Part model, mm, in its own coordinate system. Face numbers are marked on the shaded views. A direction names the side the tool comes from. Round coordinates to 2 decimals unless told otherwise and drop trailing zeros. Write each loop counter-clockwise with the first axis right and the second up, starting at its lowest first coordinate (ties: lowest second). Pieces come first, ordered by that corner, then holes. Notation, with made-up numbers: M 86.25,-31.5 L 132.25,-31.5 A25 cw 132.25,-18.5 Z; hole C -2,-3.5 d4. An arc over 180 degrees is marked long. Use a Markdown table: item, result. Add a question column.
1) Two-plate mould, pull along Y, no slides. Class the marked faces 4, 5 and 6: released by +Y, released by -Y, zero draft, split by the parting line, or undercut.
2) Wall check: probe 1 along Z at (x, y) = (-10.75, 13); probe 2 along Y at (x, z) = (9.25, 10); probe 3 along Y at (x, z) = (12.25, -13). Give the ranges that are in metal, low to high.
3) Slice it at B-B on y = 26.5. Write the cut outline in (x, z), plus the area to 3 significant figures.
4) Slice it at A-A on x = 11. Write the cut outline in (y, z).
5) Drop flat-ended pins along their axis: P1, Ø4.5, axis at x = -2, y = 7, coming from the -Z side; P2, Ø1.7, axis at x = 11, z = 16.5, coming from the +Y side; P3, Ø8.5, axis at x = -3.5, y = 20.5, coming from the +Z side. Give the stop position or say it passes through.
6) Which spindle directions (+Z, -Z, +X, -X, +Y, -Y) get a long thin tool onto all of the face, cutting with end or side? Do the marked faces 1, 2 and 3. Say none if no direction does.
7) Slice it at C-C on x = -2.75. Write the cut outline in (y, z).
Autodesk Inventor part; units mm, degrees
ref_plane "YZ Plane" through (0, 0, 0) normal (1, 0, 0) x (0, 1, 0)
ref_plane "XZ Plane" through (0, 0, 0) normal (0, 1, 0) x (-1, 0, 0)
ref_plane "XY Plane" through (0, 0, 0) normal (0, 0, 1) x (1, 0, 0)
sketch "Sketch1" plane through (0, 0, 0) normal (0, 1, 0) x (-1, 0, 0)
  line L0 (6.2884, 19.9233) -> (-5.9116, 19.9233)
  line L1 (-5.9116, 19.9233) -> (-5.9116, 12.6233)
  line L2 (-5.9116, 12.6233) -> (6.2884, 12.6233)
  line L3 (6.2884, 12.6233) -> (6.2884, 19.9233)
  point P0 (0, 0)
  dimension "d0" = 7.3
  dimension "d1" = 12.2
extrude "Extrusion1" add sketch "Sketch1" along normal blind 3
sketch "Sketch2" plane through (0, 3, 0) normal (0, 1, 0) x (1, 0, 0)
  line L0 (5.9116, -19.9233) -> (5.9116, -12.6233)
  line L1 (5.9116, -12.6233) -> (-6.2884, -12.6233)
  line L2 (-6.2884, -12.6233) -> (-6.2884, -19.9233)
  line L3 (-6.2884, -19.9233) -> (5.9116, -19.9233)
  line L4 (5.9116, -12.6233) -> (-6.2884, -12.6233)
  line L5 (-6.2884, -12.6233) -> (-6.2884, -14.1233)
  line L6 (-6.2884, -14.1233) -> (5.9116, -14.1233)
  line L7 (5.9116, -14.1233) -> (5.9116, -12.6233)
  point P0 (0, 0)
  point P1 (5.9116, -14.1233)
  dimension "d4" = 1.5
extrude "Extrusion2" add sketch "Sketch2" along normal blind 15.7 contours L6 L2 L1 L0
sketch "Sketch3" plane through (5.9116, 0, 12.6233) normal (0, 0, -1) x (-1, 0, 0)
  line L0 (0, 0) -> (12.2, 0)
  line L1 (12.2, 0) -> (12.2, 18.7)
  line L2 (0, 18.7) -> (12.2, 18.7)
  line L3 (0, 0) -> (0, 18.7)
  line L4 (0, 18.7) -> (12.2, 18.7)
  line L5 (12.2, 18.7) -> (12.2, 15.7)
  line L6 (12.2, 15.7) -> (0, 15.7)
  line L7 (0, 15.7) -> (0, 18.7)
  point P0 (5.9116, 0)
  point P1 (0, 15.7)
  dimension "d7" = 3
extrude "Extrusion3" add sketch "Sketch3" along normal blind 23.8 contours L3 L2 L1 L6
sketch "Sketch4" plane through (-6.2884, 15.7, 12.6233) normal (0, -1, 0) x (1, 0, 0)
  line L0 (0, 0) -> (12.2, 0)
  line L1 (0, 0) -> (0, -23.8)
  line L2 (12.2, -23.8) -> (0, -23.8)
  line L3 (12.2, 0) -> (12.2, -23.8)
  line L4 (12.2, -23.8) -> (0, -23.8)
  line L5 (0, -23.8) -> (0, -22.3)
  line L6 (0, -22.3) -> (12.2, -22.3)
  line L7 (12.2, -22.3) -> (12.2, -23.8)
  point P0 (6.2884, -12.6233)
  dimension "d10" = 1.5
extrude "Extrusion4" add sketch "Sketch4" along normal up to surface (15.7 mm away) contours L6 L3 L2 L1
sketch "Sketch5" plane through (5.9116, 0, -11.1767) normal (0, 0, -1) x (-1, 0, 0)
  line L0 (12.2, 18.7) -> (12.2, 0)
  line L1 (12.2, 18.7) -> (0, 18.7)
  line L2 (0, 18.7) -> (0, 0)
  line L3 (12.2, 0) -> (0, 0)
  line L4 (12.2, 0) -> (0, 0)
  line L5 (0, 0) -> (0, 3)
  line L6 (0, 3) -> (12.2, 3)
  line L7 (12.2, 3) -> (12.2, 0)
  point P0 (5.9116, 0)
  dimension "d13" = 3
extrude "Extrusion5" add sketch "Sketch5" along normal blind 5.8 contours L0 L3 L2 L6
sketch "Sketch6" plane through (0, 0, 0) normal (0, -1, 0) x (1, 0, 0)
  arc A0 (-0.7384, -2.4741) -> (0.3616, -2.4741) centre (-0.1884, -3.4267) ccw construction
  circle A1 centre (-0.1884, -3.4267) radius 1.1 construction
  arc A2 (0.3616, -32.1794) -> (-0.7384, -32.1794) centre (-0.1884, -31.2267) ccw
  circle A3 centre (-0.1884, -31.2267) radius 1.5
  circle A4 centre (-0.1884, -3.4267) radius 1.5
  point P0 (0, 0)
  dimension "d16" = 3
  dimension "d17" = 3
extrude "Extrusion6" cut sketch "Sketch6" against normal up to surface (3 mm away)
sketch "Sketch8" plane through (5.9116, 0, 19.9233) normal (1, 0, 0) x (0, 0, -1)
  line L0 (0, 0) -> (7.3, 0)
  line L1 (7.3, 0) -> (7.3, 15.7)
  line L2 (7.3, 15.7) -> (29.6, 15.7)
  line L3 (29.6, 15.7) -> (29.6, 0)
  line L4 (36.9, 0) -> (29.6, 0)
  line L5 (36.9, 3) -> (36.9, 0)
  line L6 (31.1, 3) -> (36.9, 3)
  line L7 (31.1, 18.7) -> (31.1, 3)
  line L8 (5.8, 18.7) -> (31.1, 18.7)
  line L9 (5.8, 3) -> (5.8, 18.7)
  line L10 (0, 3) -> (5.8, 3)
  line L11 (0, 0) -> (0, 3)
  line L12 (0, 0) -> (36.9, 0)
  line L13 (36.9, 0) -> (36.9, 6)
  line L14 (36.9, 6) -> (0, 6)
  line L15 (0, 6) -> (0, 0)
  point P0 (19.9233, 0)
  dimension "d22" = 6
extrude "Extrusion8" add sketch "Sketch8" along normal blind 8 contours L11 L10 L9 L14 L1 L0 | L1 L14 L3 L12 | L15 L14 L9 L10 | L3 L14 L7 L6 L5 L4 | L14 L13 L6 L7
sketch "Sketch9" plane through (-6.2884, 0, 12.6233) normal (-1, 0, 0) x (0, 0, 1)
  line L0 (-29.6, 6) -> (7.3, 6)
  line L1 (7.3, 6) -> (7.3, 0)
  line L2 (7.3, 0) -> (-29.6, 0)
  line L3 (-29.6, 0) -> (-29.6, 6)
  point P0 (-12.6233, 0)
  point P1 (7.3, 6)
  point P2 (-29.6, 0)
extrude "Extrusion9" add sketch "Sketch9" along normal blind 8
sketch "Sketch10" plane through (13.9116, 0, 19.9233) normal (1, 0, 0) x (0, 0, -1)
  line L0 (0, 6) -> (0, 0)
  line L1 (0, 0) -> (36.9, 0)
  line L2 (36.9, 0) -> (36.9, 6)
  line L3 (36.9, 6) -> (0, 6)
  line L4 (0, 6) -> (36.9, 0) construction
  line L5 (36.9, 6) -> (0, 0) construction
  circle A0 centre (18.45, 3) radius 1.5
  point P0 (19.9233, 0)
  dimension "d27" = 3
extrude "Extrusion10" cut sketch "Sketch10" against normal blind 8 contours A0
sketch "Sketch11" plane through (0, 18.7, 0) normal (0, 1, 0) x (1, 0, 0)
  line L0 (5.9116, -14.1233) -> (5.9116, 11.1767)
  line L1 (-6.2884, 11.1767) -> (5.9116, 11.1767)
  line L2 (-6.2884, -14.1233) -> (-6.2884, 11.1767)
  line L3 (-6.2884, -14.1233) -> (5.9116, -14.1233)
  line L4 (5.9116, -14.1233) -> (0, -14.1233)
  line L5 (0, -14.1233) -> (0, 11.1767)
  line L6 (0, 11.1767) -> (5.9116, 11.1767)
  line L7 (5.9116, 11.1767) -> (5.9116, -14.1233)
  point P0 (0, 0)
extrude "Extrusion11" add sketch "Sketch11" along normal blind 10 contours L3 L5 L1 L0
sketch "Sketch12" plane through (5.9116, 15.7, 12.6233) normal (1, 0, 0) x (0, 0, -1)
  line L0 (22.3, -9.7) -> (23.8, -9.7)
  line L1 (23.8, -9.7) -> (23.8, 13)
  line L2 (-1.5, 13) -> (23.8, 13)
  line L3 (-1.5, -9.7) -> (-1.5, 13)
  line L4 (-1.5, -9.7) -> (0, -9.7)
  line L5 (0, -9.7) -> (0, 0)
  line L6 (0, 0) -> (22.3, 0)
  line L7 (22.3, 0) -> (22.3, -9.7)
  line L8 (-1.5, 13) -> (23.8, 13)
  line L9 (23.8, 13) -> (23.8, 5)
  line L10 (23.8, 5) -> (-1.5, 5)
  line L11 (-1.5, 5) -> (-1.5, 13)
  point P0 (12.6233, -15.7)
  point P1 (-1.5, 5)
  dimension "d32" = 8
extrude "Extrusion12" add sketch "Sketch12" along normal up to surface (8 mm away) contours L10 L3 L2 L1
sketch "Sketch14" plane through (0, 28.7, 0) normal (0, 1, 0) x (1, 0, 0)
  line L0 (5.9116, 11.1767) -> (5.9116, -14.1233)
  line L1 (0, -14.1233) -> (13.9116, -14.1233)
  line L2 (13.9116, -14.1233) -> (13.9116, 11.1767)
  line L3 (0, 11.1767) -> (13.9116, 11.1767)
  line L4 (0, 11.1767) -> (0, -14.1233)
  line L5 (0, 11.1767) -> (13.9116, 11.1767)
  line L6 (13.9116, 11.1767) -> (13.9116, -14.1233)
  line L7 (13.9116, -14.1233) -> (0, -14.1233)
  line L8 (0, -14.1233) -> (0, 11.1767)
  point P0 (0, 0)
extrude "Extrusion14" add sketch "Sketch14" along normal blind 8
sketch "Sketch16" plane through (5.9116, 15.7, 12.6233) normal (1, 0, 0) x (0, 0, -1)
  line L0 (23.8, 5) -> (-1.5, 5)
  line L1 (-1.5, -9.7) -> (-1.5, 5)
  line L2 (-1.5, -9.7) -> (0, -9.7)
  line L3 (0, -9.7) -> (0, 0)
  line L4 (0, 0) -> (22.3, 0)
  line L5 (22.3, 0) -> (22.3, -9.7)
  line L6 (22.3, -9.7) -> (23.8, -9.7)
  line L7 (23.8, -9.7) -> (23.8, 5)
  point P0 (12.6233, -15.7)
extrude "Extrusion16" add sketch "Sketch16" along normal blind 8
sketch "Sketch17" plane through (13.9116, 0, 19.9233) normal (1, 0, 0) x (0, 0, -1)
  circle A0 centre (18.45, 3) radius 1.5
  line L0 (18.45, 3) -> (18.45, 26.5)
  circle A1 centre (18.45, 26.5) radius 1.5
  point P0 (19.9233, 0)
  dimension "d46" = 23.5
  dimension "d47" = 3
extrude "Extrusion17" cut sketch "Sketch17" against normal blind 8 contours A1
sketch "Sketch18" plane through (0, 18.7, -11.1767) normal (-1, 0, 0) x (0, 0, 1)
  line L0 (25.3, 0) -> (0, 0)
  line L1 (25.3, 0) -> (25.3, 18)
  line L2 (0, 18) -> (25.3, 18)
  line L3 (0, 0) -> (0, 18)
  line L4 (0, -12.7) -> (1.5, -12.7)
  line L5 (1.5, -3) -> (1.5, -12.7)
  line L6 (23.8, -3) -> (1.5, -3)
  line L7 (23.8, -12.7) -> (23.8, -3)
  line L8 (23.8, -12.7) -> (25.3, -12.7)
  line L9 (25.3, -12.7) -> (25.3, 0)
  line L10 (25.3, 0) -> (0, 0)
  line L11 (0, 0) -> (0, -12.7)
  point P0 (11.1767, -18.7)
extrude "Extrusion18" add sketch "Sketch18" along normal up to surface (14.2884 mm away) contours L0 L3 L2 L1
sketch "Sketch19" plane through (-6.2884, 15.7, -9.6767) normal (-1, 0, 0) x (0, 0, 1)
  line L0 (-1.5, -9.7) -> (0, -9.7)
  line L1 (0, 0) -> (0, -9.7)
  line L2 (22.3, 0) -> (0, 0)
  line L3 (22.3, -9.7) -> (22.3, 0)
  line L4 (22.3, -9.7) -> (23.8, -9.7)
  line L5 (23.8, -9.7) -> (23.8, 3)
  line L6 (23.8, 3) -> (-1.5, 3)
  line L7 (-1.5, 3) -> (-1.5, -9.7)
  point P0 (9.6767, -15.7)
extrude "Extrusion19" add sketch "Sketch19" along normal up to surface (8 mm away)
sketch "Sketch20" plane through (-14.2884, 0, 12.6233) normal (-1, 0, 0) x (0, 0, 1)
  line L0 (-23.8, 6) -> (-29.6, 6)
  line L1 (-29.6, 6) -> (-29.6, 0)
  line L2 (-29.6, 0) -> (7.3, 0)
  line L3 (7.3, 0) -> (7.3, 6)
  line L4 (7.3, 6) -> (1.5, 6)
  line L5 (1.5, 36.7) -> (1.5, 6)
  line L6 (-23.8, 36.7) -> (1.5, 36.7)
  line L7 (-23.8, 6) -> (-23.8, 36.7)
  line L8 (-22.3, 15.7) -> (-22.3, 6)
  line L9 (0, 15.7) -> (-22.3, 15.7)
  line L10 (0, 6) -> (0, 15.7)
  line L11 (0, 6) -> (-22.3, 6)
  line L12 (-29.6, 6) -> (7.3, 0) construction
  line L13 (7.3, 6) -> (-29.6, 0) construction
  circle A0 centre (-11.15, 3) radius 1.5
  point P0 (-12.6233, 0)
  dimension "d54" = 3
extrude "Extrusion20" cut sketch "Sketch20" against normal blind 8 contours A0
sketch "Sketch21" plane through (-14.2884, 0, 12.6233) normal (-1, 0, 0) x (0, 0, 1)
  circle A0 centre (-11.15, 26.5) radius 1.5
  point P0 (-12.6233, 0)
extrude "Extrusion21" cut sketch "Sketch21" against normal blind 8
sketch "Sketch22" plane through (0, 0, 0) normal (0, -1, 0) x (1, 0, 0)
  arc A0 (0.3616, -13.4794) -> (-0.7384, -13.4794) centre (-0.1884, -12.5267) ccw
  arc A1 (-0.7384, 16.2259) -> (0.3616, 16.2259) centre (-0.1884, 15.2733) ccw
  circle A2 centre (-0.1884, 15.2733) radius 1.5
  circle A3 centre (-0.1884, -12.5267) radius 1.5
  point P0 (0, 0)
  dimension "d59" = 3
  dimension "d60" = 3
extrude "Extrusion22" cut sketch "Sketch22" against normal blind 15
properties part number "support servo"
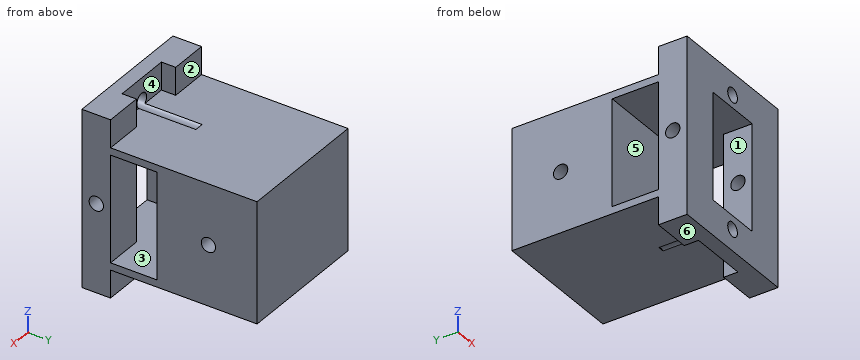
Entries:
| question | item | result |
|---|---|---|
| 1 | face 4 | released by +Y |
| 1 | face 5 | undercut |
| 1 | face 6 | zero draft |
| 2 | probe 1 | z = -11.18 to -9.68, 12.62 to 14.12 |
| 2 | probe 2 | y = 0 to 6, 15.7 to 36.7 |
| 2 | probe 3 | y = 0 to 6 |
| 3 | outline | M -14.29,-11.18 L 13.91,-11.18 L 13.91,-0.03 L 5.91,-0.03 L 5.91,2.97 L 13.91,2.97 L 13.91,14.12 L -14.29,14.12 L -14.29,2.97 L -6.29,2.97 L -6.29,-0.03 L -14.29,-0.03 Z |
| 3 | area | 665 mm^2 |
| 4 | outline | M 0,-16.98 L 6,-16.98 L 6,-11.18 L 36.7,-11.18 L 36.7,14.12 L 6,14.12 L 6,19.92 L 0,19.92 Z; hole C 3,1.47 d3; hole M 6,-9.68 L 15.7,-9.68 L 15.7,12.62 L 6,12.62 Z; hole C 26.5,1.47 d3 |
| 5 | P1 | stops at z = -11.18 |
| 5 | P2 | stops at y = 6 |
| 5 | P3 | stops at z = 14.12 |
| 6 | face 1 | -Y |
| 6 | face 2 | +Z, +X, -X, +Y |
| 6 | face 3 | none |
| 7 | outline | M 0,-16.98 L 3,-16.98 L 3,-11.18 L 36.7,-11.18 L 36.7,14.12 L 3,14.12 L 3,19.92 L 0,19.92 L 0,12.62 L 15.7,12.62 L 15.7,-9.68 L 0,-9.68 Z |
